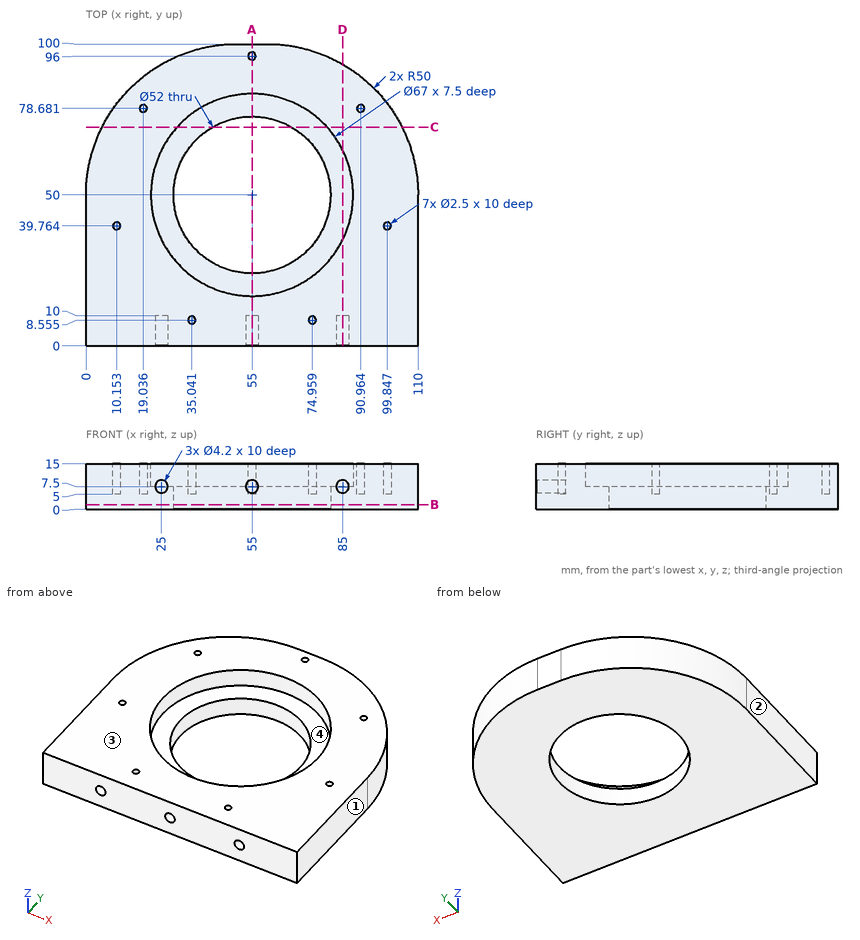
Check sheet for the drawn part. Datum: minimum x, y, z corner. Units: mm. Give positions to 0.01 mm unless a question says otherwise; leave off trailing zeros. Order: outer loops, then holes, each group sorted by start corner. A loop starts at its lowest first (then second) coordinate and runs counter-clockwise, first axis right, second up. Notation, with made-up numbers: (10, 79.25) - (44, 79.25) arc R13 cw to (44, 91.25) - close; hole circle Ø5 at (47.5, 86). An arc over 180 degrees is marked (long way). Answer as a JSON object with one key per item and string values.
(1) Depth check by flat-ended pin: pin 1 Ø4 at (y, z) = (60.5, 11) entering from -X; pin 2 Ø4 at (y, z) = (78, 7) entering from -X; pin 3 Ø2 at (x, y) = (90.96, 78.68) entering from +Z. Enter the tip coordinate at first touch or a pass-through.
Report:
{"pin 1": "x = 0.73", "pin 2": "x = 7.29", "pin 3": "z = 5"}
(2) Cross-section at D-D (x = 85). Record the cut outline in (y, z), then the cut area to 3 significant figures.
Report:
{"outline": "(0, 0) - (93.3, 0) - (93.3, 15) - (64.91, 15) - (64.91, 7.5) - (35.09, 7.5) - (35.09, 15) - (0, 15) - (0, 9.6) - (10, 9.6) - (10, 5.4) - (0, 5.4) - close", "area": "1,130 mm^2"}
(3) Cross-section at C-C (y = 72.5). Record the cut outline in (x, z).
Report:
{"outline": "(5.35, 0) - (41.97, 0) - (41.97, 7.5) - (30.18, 7.5) - (30.18, 15) - (5.35, 15) - close; (68.03, 0) - (104.65, 0) - (104.65, 15) - (79.82, 15) - (79.82, 7.5) - (68.03, 7.5) - close"}
(4) Material ranges on line 1 (Y direction, x = 55, z = 9.75); line 2 (X direction, y = 6, z = 8.5) (1 decimal); line 3 (X direction, y = 65.5, z = 2.75) (1 decimal), recorded low to high.
Report:
{"line 1": "0 to 16.5, 83.5 to 94.75, 97.25 to 100", "line 2": "0 to 23.2, 26.8 to 53.2, 56.8 to 83.2, 86.8 to 110", "line 3": "2.5 to 34.1, 75.9 to 107.5"}
(5) Cross-section at A-A (x = 55). Record the cut outline in (y, z).
Report:
{"outline": "(0, 0) - (24, 0) - (24, 7.5) - (16.5, 7.5) - (16.5, 15) - (0, 15) - (0, 9.6) - (10, 9.6) - (10, 5.4) - (0, 5.4) - close; (76, 0) - (100, 0) - (100, 15) - (97.25, 15) - (97.25, 5) - (94.75, 5) - (94.75, 15) - (83.5, 15) - (83.5, 7.5) - (76, 7.5) - close"}
(6) Draft check along X on the marked faces 1, 2, 3 and 4. Enter one of: released by +X, released by -X, zero draft, split by the parting line, or undercut.
Report:
{"face 1": "released by +X", "face 2": "released by -X", "face 3": "zero draft", "face 4": "undercut"}
(7) Cross-section at B-B (z = 1.5). Record the cut outline in (x, y).
Report:
{"outline": "(0, 0) - (110, 0) - (110, 50) arc R50 ccw to (60, 100) - (50, 100) arc R50 ccw to (0, 50) - close; hole circle Ø52 at (55, 50)"}
